The listing builds one solid part. Answer for the finished solid, in the listing's coordinates (mm). A direction names the side the tool comes from. Coordinates: 2 decimals unless noted, no trailing zeros. Order: outer loops, then holes, each group sorted by start corner. A loop starts at its lowest first (then second) coordinate and runs counter-clockwise, first axis right, second up. Notation, with made-up numbers: (-16, -10) -> (31, -10) arc R17 cw to (31, -1) -> close; hole circle Ø2 at (75.25, -9). An arc over 180 degrees is marked (long way). Write item = value, one per line.
from build123d import *

# Parameters (mm, degrees)
F1_DEPTH       = 65
F2_SIZE        = 5
F5_D           = 6.6
F5_CBORE_D     = 11.25
F5_CBORE_DEPTH = 7
F6_D           = 5.5
F6_DEPTH       = 4.5
F6_TIP         = 1.6523667023
F8_DEPTH       = 37
F10_DEPTH      = 26


with BuildPart() as f1:
    # F0 (on Front) → F1 (new body)
    with BuildSketch(Plane.XZ):
        Polygon((45.5, -13.25), (45.5, 13.25), (35, 13.25), (38.7527767497, 6.75), (21.25, 6.75), (25.147114317, 0), (0, 0), (-25.147114317, 0), (-21.25, 6.75), (-38.7527767497, 6.75), (-35, 13.25), (-45.5, 13.25), (-45.5, -13.25), align=None)
    extrude(amount=F1_DEPTH)

    # F2
    f2_edges = [f1.edges().sort_by_distance(p)[0] for p in [
        (45.5, -65, 0),
        (45.5, 0, 0),
        (-45.5, -65, 0),
        (-45.5, 0, 0),
    ]]
    chamfer(f2_edges, length=F2_SIZE)

    # F5 (through all)
    with Locations(Plane.XY):
        with Locations((9.9724601813, -22.4858294427), (-10.0275398187, -22.4858294427), (-10.0275398187, -42.4858294427), (9.9724601813, -42.4858294427), (-0.0275398187, -32.4858294427)):
            CounterBoreHole(F5_D / 2, F5_CBORE_D / 2, F5_CBORE_DEPTH)

    # F6
    with Locations(Plane(origin=(0, 0, -13.25), x_dir=(1, 0, 0), z_dir=(0, 0, -1))):
        with Locations((27, 32.5), (20, 22.5), (20, 42.5), (-10, 5), (-10, 60)):
            Hole(F6_D / 2, depth=F6_DEPTH)
            with Locations((0, 0, -(F6_DEPTH + F6_TIP / 2))):  # 118° drill point
                Cone(0, F6_D / 2, F6_TIP, mode=Mode.SUBTRACT)



with BuildPart() as f8:
    # F7 (on face) → F8 (new body)
    with BuildSketch(Plane(origin=(-45.5, 0, 0), x_dir=(0, -1, 0), z_dir=(-1, 0, 0))):
        with BuildLine():
            ThreePointArc((35.0980762114, -13.25), (38.2959698705, -10.6751411771), (39.5, -6.75))
            ThreePointArc((39.5, -6.75), (28.5748588229, -0.9540301295), (29.9019237886, -13.25))
            Line((29.9019237886, -13.25), (35.0980762114, -13.25))
        make_face()
    extrude(amount=F8_DEPTH)


with BuildPart() as f1_1:
    add(f1.part)

    add(f8.part)  # F10 merges F8
    # F9 (on face) → F10 (join)
    with BuildSketch(Plane(origin=(-82.5, 0, 0), x_dir=(0, -1, 0), z_dir=(-1, 0, 0))):
        with BuildLine():
            ThreePointArc((42.4532659811, -7.7156584847), (42.4883096621, -7.2333943467), (42.5, -6.75))
            ThreePointArc((42.5, -6.75), (42.4883096621, -6.2666056533), (42.4532659811, -5.7843415153))
            ThreePointArc((42.4532659811, -5.7843415153), (40.9160983506, -4.0154438804), (41.1199611443, -1.680851169))
            ThreePointArc((41.1199611443, -1.680851169), (40.5901699437, -0.8721474771), (39.9847615122, -0.1183829193))
            ThreePointArc((39.9847615122, -0.1183829193), (37.7014348334, 0.4091608651), (36.4941241321, 2.4177135872))
            ThreePointArc((36.4941241321, 2.4177135872), (35.5901699437, 2.760565163), (34.6573325433, 3.0145233523))
            ThreePointArc((34.6573325433, 3.0145233523), (32.5, 2.0992094912), (30.3426674567, 3.0145233523))
            ThreePointArc((30.3426674567, 3.0145233523), (29.4098300563, 2.760565163), (28.5058758679, 2.4177135872))
            ThreePointArc((28.5058758679, 2.4177135872), (27.2985651666, 0.4091608651), (25.0152384878, -0.1183829193))
            ThreePointArc((25.0152384878, -0.1183829193), (24.4098300563, -0.8721474771), (23.8800388557, -1.680851169))
            ThreePointArc((23.8800388557, -1.680851169), (24.141738822, -2.3631068384), (24.2307321005, -3.0883928973))
            ThreePointArc((24.2307321005, -3.0883928973), (23.775138294, -4.6777314775), (22.5467340189, -5.7843415153))
            ThreePointArc((22.5467340189, -5.7843415153), (22.5, -6.75), (22.5467340189, -7.7156584847))
            ThreePointArc((22.5467340189, -7.7156584847), (23.775138294, -8.8222685225), (24.2307321005, -10.4116071027))
            ThreePointArc((24.2307321005, -10.4116071027), (24.141738822, -11.1368931616), (23.8800388557, -11.819148831))
            ThreePointArc((23.8800388557, -11.819148831), (24.4098300563, -12.6278525229), (25.0152384878, -13.3816170807))
            ThreePointArc((25.0152384878, -13.3816170807), (27.2985651666, -13.9091608651), (28.5058758679, -15.9177135872))
            ThreePointArc((28.5058758679, -15.9177135872), (29.4098300563, -16.260565163), (30.3426674567, -16.5145233523))
            ThreePointArc((30.3426674567, -16.5145233523), (32.5, -15.5992094912), (34.6573325433, -16.5145233523))
            ThreePointArc((34.6573325433, -16.5145233523), (35.5901699437, -16.260565163), (36.4941241321, -15.9177135872))
            ThreePointArc((36.4941241321, -15.9177135872), (37.7014348334, -13.9091608651), (39.9847615122, -13.3816170807))
            ThreePointArc((39.9847615122, -13.3816170807), (40.5901699437, -12.6278525229), (41.1199611443, -11.819148831))
            ThreePointArc((41.1199611443, -11.819148831), (40.9160983506, -9.4845561196), (42.4532659811, -7.7156584847))
        make_face()
        with BuildLine():
            ThreePointArc((29.9019237886, -13.25), (32.5, 0.25), (35.0980762114, -13.25))
            Line((35.0980762114, -13.25), (29.9019237886, -13.25))
        make_face(mode=Mode.SUBTRACT)
        with BuildLine():
            Line((29.9019237886, -13.25), (35.0980762114, -13.25))
            ThreePointArc((35.0980762114, -13.25), (32.5, 0.25), (29.9019237886, -13.25))
        make_face()
    extrude(amount=-F10_DEPTH)


solid = f1_1.part
Q1. A tool of negligible diameter and unlimited length cuts with its end or side. For faces 4 (the face through (15.34, -40.8, -3.45)), 5 (the face through (-69.7, -32.5, 2.1)), 6 (the face through (23.171, -32.045, 3.422)), 7 (the face through (0.688, -35.707, -10.169)), from which of +Z, -Z, +X, -X, +Y, -Y can it reach the whole face along a straight path? Write none if from no direction.
The answers:
face_4 = +Z
face_5 = +Z, -X
face_6 = +Y, -Y
face_7 = +Z, -Z
Q2. The mould has two halves that part along Y. Classify faces 1 (the face through (43, -2.5, -0.2)), 2 (the face through (-10, -26, -7)), 3 (the face through (-30, -32, 6.75)): released by +Y, released by -Y, zero draft, split by the parting line, or undercut.
The answers:
face_1 = released by +Y
face_2 = undercut
face_3 = zero draft
Q3. Each of these flat-tipped pins is pushed along its axis until it touches: pin 1 Ø9 at (x, y) = (-0.03, -32.49) entering from -Z; pin 2 Ø1 at (x, y) = (-51.5, -37) entering from -Z; pin 3 Ø3.5 at (x, y) = (-9, -23.5) entering from +Z; pin 4 Ø6.5 at (x, y) = (20, -22.5) entering from +Z. Where does it stop, or does it pass through?
The answers:
pin_1 = -13.25
pin_2 = -12.49
pin_3 = through
pin_4 = 6.75
Q4. Section D-D, the plane x = -19 is taken. Give the vertices of the cut face in (y, z), plus the area to 3 significant figures.
The answers:
outline = (-65, -13.25) -> (0, -13.25) -> (0, 0) -> (-65, 0) -> close
area = 861 mm2
Q5. Section C-C, the plane x = 8 is taken. Give the vertices of the cut face in (y, z), plus the area to 3 significant figures.
The answers:
outline = (-65, -13.25) -> (-45.13, -13.25) -> (-45.13, -7) -> (-47.75, -7) -> (-47.75, 0) -> (-65, 0) -> close; (-39.84, -13.25) -> (-25.13, -13.25) -> (-25.13, -7) -> (-27.75, -7) -> (-27.75, 0) -> (-37.22, 0) -> (-37.22, -7) -> (-39.84, -7) -> close; (-19.84, -13.25) -> (0, -13.25) -> (0, 0) -> (-17.22, 0) -> (-17.22, -7) -> (-19.84, -7) -> close
area = 648 mm2
Q6. Section B-B, the plane z = 10 is taken. Give the vertices of the cut face in (x, y).
The answers:
outline = (-45.5, -60) -> (-40.5, -65) -> (-36.88, -65) -> (-36.88, 0) -> (-40.5, 0) -> (-45.5, -5) -> close; (36.88, -65) -> (40.5, -65) -> (45.5, -60) -> (45.5, -5) -> (40.5, 0) -> (36.88, 0) -> close
Q7. Section A-A, the plane x = -70 is taken. Give the vertices of the cut face in (y, z).
The answers:
outline = (-42.45, -7.72) arc R3 cw to (-41.12, -11.82) arc R10 ccw to (-39.98, -13.38) arc R3 cw to (-36.49, -15.92) arc R10 ccw to (-34.66, -16.51) arc R3 cw to (-30.34, -16.51) arc R10 ccw to (-28.51, -15.92) arc R3 cw to (-25.02, -13.38) arc R10 ccw to (-23.88, -11.82) arc R3 cw to (-22.55, -7.72) arc R10 ccw to (-22.55, -5.78) arc R3 cw to (-23.88, -1.68) arc R10 ccw to (-25.02, -0.12) arc R3 cw to (-28.51, 2.42) arc R10 ccw to (-30.34, 3.01) arc R3 cw to (-34.66, 3.01) arc R10 ccw to (-36.49, 2.42) arc R3 cw to (-39.98, -0.12) arc R10 ccw to (-41.12, -1.68) arc R3 cw to (-42.45, -5.78) arc R10 ccw to start
Q8. Find the intervals of material crossed by line 1 along X through (y, z) = (-32.5, -11); line 2 along X through (y, z) = (-42.5, -11.35); line 3 along X through (y, z) = (-42.5, -3), in increasing order.
The answers:
line_1 = -82.5 to -3.33, 3.27 to 24.25, 29.75 to 45.5
line_2 = -45.5 to -13.33, -6.73 to 6.67, 13.27 to 17.25, 22.75 to 45.5
line_3 = -45.5 to -15.65, -4.4 to 4.35, 15.6 to 45.5
